```python
from build123d import *

# Parameters (mm, degrees)
BOSS_EXTRUDE1_DEPTH = 76.2
CUT_EXTRUDE2_DEPTH  = 1779.906911561


with BuildPart() as part:
    # Sketch1 → Boss-Extrude1 (new body)
    with BuildSketch(Plane.XY):
        with BuildLine():
            Line((101.6, 0), (914.4, 0))
            Line((914.4, 0), (914.4, 1524))
            Line((914.4, 1524), (101.6, 1524))
            ThreePointArc((101.6, 1524), (29.757951031, 1494.242048969), (0, 1422.4))
            Line((0, 1422.4), (0, 101.6))
            ThreePointArc((0, 101.6), (29.757951031, 29.757951031), (101.6, 0))
        make_face()
    extrude(amount=BOSS_EXTRUDE1_DEPTH)

    # Sketch2 → Cut-Extrude2 (cut, through all)
    with BuildSketch(Plane.XY.offset(76.2)):
        with BuildLine():
            Line((63.5, 1422.4), (63.5, 101.6))
            ThreePointArc((63.5, 101.6), (74.659231637, 74.659231637), (101.6, 63.5))
            Line((101.6, 63.5), (850.9, 63.5))
            Line((850.9, 63.5), (850.9, 1460.5))
            Line((850.9, 1460.5), (101.6, 1460.5))
            ThreePointArc((101.6, 1460.5), (74.659231637, 1449.340768363), (63.5, 1422.4))
        make_face()
    extrude(amount=-CUT_EXTRUDE2_DEPTH, mode=Mode.SUBTRACT)


solid = part.part
```
Geometry: final body of the model. Coordinates: model frame, mm. A direction names the side the tool comes from. Coordinates: 2 decimals unless noted, no trailing zeros. Order: outer loops, then holes, each group sorted by start corner. A loop starts at its lowest first (then second) coordinate and runs counter-clockwise, first axis right, second up. Notation, with made-up numbers: (2, 59.5) - (50, 59.5) arc R19 cw to (50, 85.5) - close; hole circle Ø11 at (42, -32). An arc over 180 degrees is marked (long way). Return JSON: item names as keys, results as strings. Group by question number.
1. Pull-direction query (X, two-part tool) for faces 3 (the face through (861, 766, 0)), 4 (the face through (28.972, 30.552, 37.567)), 5 (the face through (914.4, 751, 38)), 6 (the face through (63.5, 771, 39)); classes: pulls with the +X half, pulls with the -X half, needs draft (parallel to the pull), parting line crosses it, or undercut.
2. Cut plane A-A (z = 36). Output: boundary loops of the cut face in (x, y).
3. Set-up query: faces 1 (the face through (481, 1460.5, 39)), 2 (the face through (30.552, 1495.028, 37.567)). Return all of +Z, -Z, +X, -X, +Y, -Y with unobstructed straight access to the full face (end or side cutting, diameter ignored); none if empty.
4. Cut plane C-C (y = 181). Output: boundary loops of the cut face in (x, z).
5. Material intervals for line 1 along Y through (x, z) = (297, 4); line 2 along X through (y, z) = (940.5, 58.5), sorted ascending. Write a range as [from, to].
6. Cut plane B-B (x = 255). Output: boundary loops of the cut face in (y, z), plus the area to 3 significant figures.
Resolved:
{
 "1": {"face 3": "needs draft", "face 4": "pulls with the -X half", "face 5": "pulls with the +X half", "face 6": "undercut"},
 "2": {"outline": "(0, 101.6) arc R101.6 ccw to (101.6, 0) - (914.4, 0) - (914.4, 1524) - (101.6, 1524) arc R101.6 ccw to (0, 1422.4) - close; hole (63.5, 101.6) arc R38.1 ccw to (101.6, 63.5) - (850.9, 63.5) - (850.9, 1460.5) - (101.6, 1460.5) arc R38.1 ccw to (63.5, 1422.4) - close"},
 "3": {"face 1": "+Z, -Z", "face 2": "+Z, -Z, -X, +Y"},
 "4": {"outline": "(0, 0) - (63.5, 0) - (63.5, 76.2) - (0, 76.2) - close; (850.9, 0) - (914.4, 0) - (914.4, 76.2) - (850.9, 76.2) - close"},
 "5": {"line 1": "y = [0, 63.5], [1460.5, 1524]", "line 2": "x = [0, 63.5], [850.9, 914.4]"},
 "6": {"outline": "(0, 0) - (63.5, 0) - (63.5, 76.2) - (0, 76.2) - close; (1460.5, 0) - (1524, 0) - (1524, 76.2) - (1460.5, 76.2) - close", "area": "9,680 mm²"}
}
